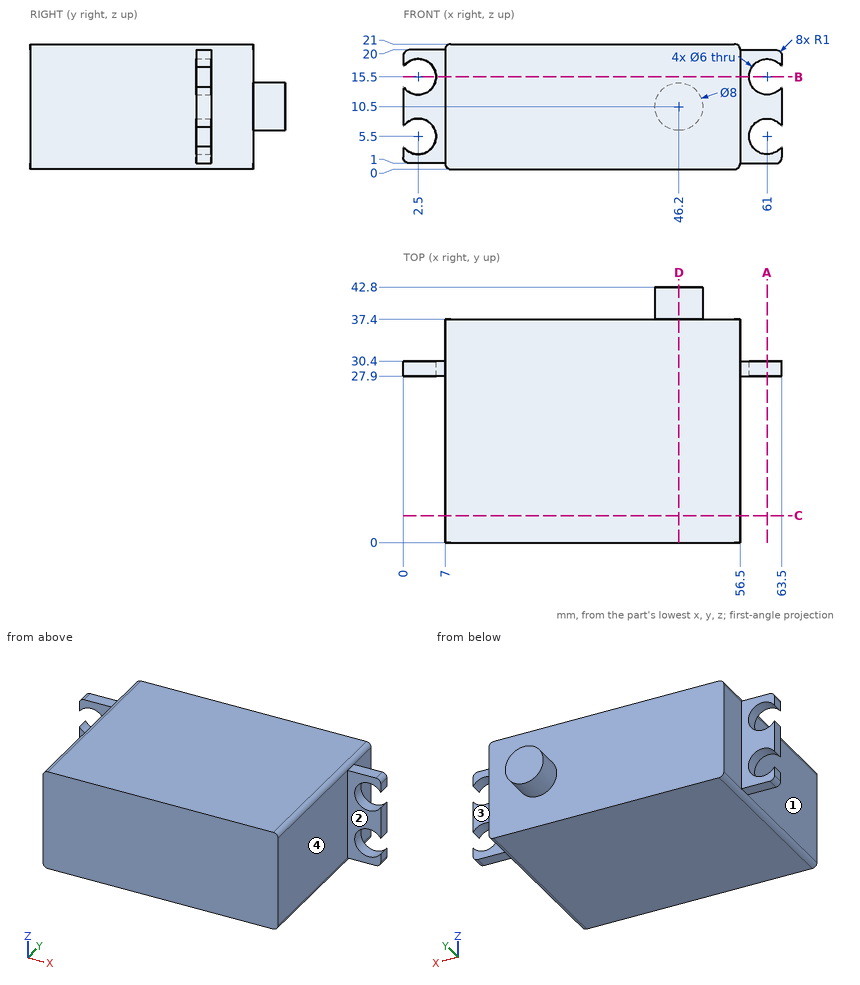
Input: dimensioned drawing with shaded views. Units: mm. Origin: part minimum x, y, z. A direction names the side the tool comes from. Coordinates: 2 decimals unless noted, no trailing zeros. Loops run counter-clockwise (first coordinate to the right, second up) from the corner with the lowest first, then second, coordinate; pieces in that order, holes last. Notation, with made-up numbers: M -19.75,58.5 L 5.25,58.5 A26 ccw 5.25,84.5 Z; hole C 32,19 d9. An arc over 180 degrees is marked long. Use a Markdown table: item, result. Add a question column.
Q1. Material intervals for L1, parallel to Z at x = 61, y = 28; L2, parallel to X at y = 29.45, z = 15.5; L3, parallel to Y at x = 26.5, z = 16.5, sorted ascending.
Q2. Section query A-A, the plane x = 61. Return loops of the section in (y, z), and give its area (3 significant figures).
Q3. Section query C-C, the plane y = 4.5. Return loops of the section in (x, z), and give its area (3 significant figures).
Q4. Access query for the marked faces 1, 2, 3 and 4. Directions: +Z, -Z, +X, -X, +Y, -Y. A direction counts if a zero-diameter tool reaches every point of the face in a straight line with its end or side. Return the directions, or none.
Q5. First-contact query: pin 1 (7.5 mm diameter, centred on x = 61.5, z = 10.5, fed in from -Y); pin 2 (1.2 mm diameter, centred on x = 59, y = 29.5, fed in from +Z); pin 3 (10 mm diameter, centred on y = 12, z = 10.5, fed in from -X). Flat tips, straight axial feed; report the tip coordinate or a pass-through.
Q6. Section query D-D, the plane x = 46.2. Return loops of the section in (y, z).
Q7. Section query B-B, the plane z = 15.5. Return loops of the section in (x, y).
Result:
| question | item | result |
|---|---|---|
| 1 | L1 | z = 1 to 2.5, 8.5 to 12.5, 18.5 to 20 |
| 1 | L2 | x = 5.5 to 58 |
| 1 | L3 | y = 0 to 37.4 |
| 2 | outline | M 27.9,1 L 30.4,1 L 30.4,2.5 L 27.9,2.5 Z; M 27.9,8.5 L 30.4,8.5 L 30.4,12.5 L 27.9,12.5 Z; M 27.9,18.5 L 30.4,18.5 L 30.4,20 L 27.9,20 Z |
| 2 | area | 17.5 mm2 |
| 3 | outline | M 7,1 A1 ccw 8,0 L 55.5,0 A1 ccw 56.5,1 L 56.5,20 A1 ccw 55.5,21 L 8,21 A1 ccw 7,20 Z |
| 3 | area | 1,040 mm2 |
| 4 | face 1 | +Z, -Z, -X, -Y |
| 4 | face 2 | +Z, -Z, +X, -Y |
| 4 | face 3 | +Z, -Z, +X, +Y |
| 4 | face 4 | +Z, -Z, +X, -Y |
| 5 | pin 1 | stops at y = 27.9 |
| 5 | pin 2 | stops at z = 20 |
| 5 | pin 3 | stops at x = 7 |
| 6 | outline | M 0,0 L 37.4,0 L 37.4,6.5 L 42.8,6.5 L 42.8,14.5 L 37.4,14.5 L 37.4,21 L 0,21 Z |
| 7 | outline | M 5.5,27.9 L 7,27.9 L 7,0 L 56.5,0 L 56.5,27.9 L 58,27.9 L 58,30.4 L 56.5,30.4 L 56.5,37.4 L 7,37.4 L 7,30.4 L 5.5,30.4 Z |
